from build123d import *
from build123d import SkipClean  # not in build123d's __all__

# Parameters (mm, degrees)
F0_R      = 11
F1_DEPTH  = 3.5
F2_R      = 5.1
F3_DEPTH  = 10
F4_R      = 4
F5_DEPTH  = 25
F6_R      = 5.1
F6_R_2    = 4
F7_DEPTH  = 1.5
F8_SIZE   = 0.5
F9_R      = 1.75
F10_DEPTH = 5.001


# Not quite as in the source:
# - after a boolean that leaves OpenCascade's solid faulty, fix() repairs it


with BuildPart() as f1:
    # F0 (on Right) → F1 (new body)
    with BuildSketch(Plane.YZ):
        Circle(F0_R)
    extrude(amount=F1_DEPTH)

    # F2 (on face) → F3 (join)
    with BuildSketch(Plane.YZ.offset(3.5)):
        Circle(F2_R)
    extrude(amount=F3_DEPTH)

    # F4 (on face) → F5 (cut)
    with BuildSketch(Plane.YZ.offset(13.5)):
        Circle(F4_R)
    extrude(amount=-F5_DEPTH, mode=Mode.SUBTRACT)

    # F6 (on face) → F7 (join)
    with BuildSketch(Plane(origin=(0, 0, 0), x_dir=(0, -1, 0), z_dir=(-1, 0, 0))):
        Circle(F6_R)
        Circle(F6_R_2, mode=Mode.SUBTRACT)
    with SkipClean():  # cleaning this boolean's faces spoils the solid; the shape is the same uncleaned
        extrude(amount=F7_DEPTH)

    # F8
    f8_edges = [f1.edges().sort_by_distance(p)[0] for p in [
        (13.5, -5.1, 0),
        (3.5, -11, 0),
        (0, -11, 0),
        (-1.5, 5.1, 0),
        (3.5, -5.1, 0),
    ]]
    chamfer(f8_edges, length=F8_SIZE)

    # F9 (on face) → F10 (cut, through all)
    with BuildSketch(Plane.YZ.offset(3.5)):
        with Locations((0, 8)):
            Circle(F9_R)
        with Locations((-8, 0)):
            Circle(F9_R)
        with Locations((0, -8)):
            Circle(F9_R)
        with Locations((8, 0)):
            Circle(F9_R)
    extrude(amount=-F10_DEPTH, mode=Mode.SUBTRACT)

    add(f1.part.fix(), mode=Mode.REPLACE)


solid = f1.part
Geometry check sheet. Reference: the model listing, model coordinates, mm. A direction names the side the tool comes from. Round coordinates to 2 decimals unless told otherwise and drop trailing zeros. Order: outer loops, then holes, each group sorted by start corner. A loop starts at its lowest first (then second) coordinate and runs counter-clockwise, first axis right, second up. Notation, with made-up numbers: M 64.25,75 L 78.25,75 A22 cw 78.25,92 Z; hole C 87.5,56 d5. An arc over 180 degrees is marked long. Answer in a Markdown table with one row per item. Add a question column.
Item 1: Draft check along Y on faces 3 (the face through (1.774, -0.228, 9.735)), 4 (the face through (3.5, 5, -5)), 5 (the face through (1.774, 9.669, 0.526)), 6 (the face through (8.4, 2.4, -4.5)). Enter one of: released by +Y, released by -Y, zero draft, split by the parting line, or undercut.
Item 2: Sectioned sample at C-C, the plane x = 8.75. Enter the section's corners in (y, z).
Item 3: Set-up check for faces 1 (the face through (-0.5, -2.4, -4.5)), 2 (the face through (-1.5, 1.7, 3.8)): record each of +Z, -Z, +X, -X, +Y, -Y from which the full face is reachable in a straight line by a thin tool's end or side.
Item 4: Material ranges on L1, parallel to X at y = 5.5, z = 8; L2, parallel to Z at x = 3.75, y = -2.25; L3, parallel to Z at x = 1.75, y = -8.5, recorded low to high. Write a range as [from, to].
Item 5: Sectioned sample at A-A, the plane z = 0. State how many separate pieces and enclosed holes the cut face has, plus the area to 4 significant figures.
Item 6: Depth check by flat-ended pin: pin 1 Ø5 at (y, z) = (0, 0) entering from -X; pin 2 Ø8 at (x, y) = (5, -7.5) entering from +Z; pin 3 Ø1.5 at (y, z) = (-7, 7.5) entering from +X; pin 4 Ø6 at (x, z) = (9.5, 4.5) entering from +Y. Enter the tip coordinate at first touch or a pass-through.
Filled in:
| question | item | result |
|---|---|---|
| 1 | face 3 | undercut |
| 1 | face 4 | zero draft |
| 1 | face 5 | undercut |
| 1 | face 6 | split by the parting line |
| 2 | outline | C 0,0 d10.2; hole C 0,0 d8 |
| 3 | face 1 | -X |
| 3 | face 2 | +Z, -Z, -X, +Y, -Y |
| 4 | L1 | x = [0, 3.5] |
| 4 | L2 | z = [-4.85, -3.31], [3.31, 4.85] |
| 4 | L3 | z = [-6.98, -1.68], [1.68, 6.98] |
| 5 | separate pieces | 4 |
| 5 | enclosed holes | 0 |
| 5 | area | 49.05 mm² |
| 6 | pin 1 | passes through |
| 6 | pin 2 | stops at z = 10.23 |
| 6 | pin 3 | stops at x = 3.5 |
| 6 | pin 4 | stops at y = 4.87 |
